from build123d import *

# Parameters (mm, degrees)
BOSS_EXTRUDE1_DEPTH   = 90
BOSS_EXTRUDE1_2_DEPTH = 90
SKETCH3_W             = 2
SKETCH3_H             = 3.026273801
EXTRUDE_THIN1_DEPTH   = 160
SKETCH5_W             = 160
SKETCH5_H             = 110
BOSS_EXTRUDE2_DEPTH   = 5
BOSS_EXTRUDE3_DEPTH   = 5
SKETCH7_W             = 2
SKETCH7_H             = 100
CUT_EXTRUDE1_DEPTH    = 2.5
SKETCH8_W             = 2
SKETCH8_H             = 90
CUT_EXTRUDE2_DEPTH    = 2.5
SKETCH9_W             = 2
SKETCH9_H             = 90
CUT_EXTRUDE3_DEPTH    = 2.5
SKETCH10_W            = 2
SKETCH10_H            = 2.5
CUT_EXTRUDE4_DEPTH    = 2.5
BOSS_EXTRUDE4_DEPTH   = 160
SKETCH12_W            = 100
SKETCH12_H            = 110
BOSS_EXTRUDE5_DEPTH   = 5
FILLET1_R             = 1


with BuildPart() as part:
    # Sketch2 → Boss-Extrude1 (new body)
    with BuildSketch(Plane.XY):
        Polygon((80, 55), (-80, 55), (-80, 50), (-75, 50), (75, 50), (80, 50), align=None)
    extrude(amount=BOSS_EXTRUDE1_DEPTH)



with BuildPart() as body_2:
    # Sketch2 → Boss-Extrude1 2 (new body)
    with BuildSketch(Plane.XY):
        Polygon((-75, -50), (-80, -50), (-80, -55), (80, -55), (80, -50), (75, -50), align=None)
    extrude(amount=BOSS_EXTRUDE1_2_DEPTH)


with BuildPart() as part_1:
    add(part.part)

    add(body_2.part)  # Extrude-Thin1 merges body 2
    # Sketch3 → Extrude-Thin1 (add)
    with BuildSketch(Plane(origin=(80, 0, 0), x_dir=(0, 0, -1), z_dir=(1, 0, 0))):
        with Locations((-36, 48.486863099)):
            Rectangle(SKETCH3_W, SKETCH3_H)
        with Locations((-34, -48.486863099)):
            Rectangle(SKETCH3_W, SKETCH3_H)
        with Locations((-40, 48.486863099)):
            Rectangle(SKETCH3_W, SKETCH3_H)
        with Locations((-38, -48.486863099)):
            Rectangle(SKETCH3_W, SKETCH3_H)
    extrude(amount=-EXTRUDE_THIN1_DEPTH)

    # Sketch5 → Boss-Extrude2 (add)
    with BuildSketch(Plane(origin=(0, 0, 0), x_dir=(-1, 0, 0), z_dir=(0, 0, -1))):
        Rectangle(SKETCH5_W, SKETCH5_H)
    extrude(amount=BOSS_EXTRUDE2_DEPTH)

    # Sketch6 → Boss-Extrude3 (add)
    with BuildSketch(Plane(origin=(80, 0, 0), x_dir=(0, 0, -1), z_dir=(1, 0, 0))):
        Polygon((-90, 55), (-90, 50), (0, 50), (0, -50), (-90, -50), (-90, -55), (5, -55), (5, 55), align=None)
    extrude(amount=BOSS_EXTRUDE3_DEPTH)

    # Sketch7 → Cut-Extrude1 (cut)
    with BuildSketch(Plane.XY):
        with Locations((82.5, 0)):
            Rectangle(SKETCH7_W, SKETCH7_H)
    extrude(amount=-CUT_EXTRUDE1_DEPTH, mode=Mode.SUBTRACT)

    # Sketch8 → Cut-Extrude2 (cut)
    with BuildSketch(Plane.XZ.offset(-50)):
        with Locations((82.5, 45)):
            Rectangle(SKETCH8_W, SKETCH8_H)
    extrude(amount=-CUT_EXTRUDE2_DEPTH, mode=Mode.SUBTRACT)

    # Sketch9 → Cut-Extrude3 (cut)
    with BuildSketch(Plane(origin=(0, -50, 0), x_dir=(1, 0, 0), z_dir=(0, 1, 0))):
        with Locations((82.5, -45)):
            Rectangle(SKETCH9_W, SKETCH9_H)
    extrude(amount=-CUT_EXTRUDE3_DEPTH, mode=Mode.SUBTRACT)

    # Sketch10 → Cut-Extrude4 (cut)
    with BuildSketch(Plane.XY):
        with Locations((82.5, 51.25)):
            Rectangle(SKETCH10_W, SKETCH10_H)
        with Locations((82.5, -51.25)):
            Rectangle(SKETCH10_W, SKETCH10_H)
    extrude(amount=-CUT_EXTRUDE4_DEPTH, mode=Mode.SUBTRACT)

    # Sketch11 → Boss-Extrude4 (add)
    with BuildSketch(Plane.ZY.offset(80)):
        Polygon((90, 50), (90, 55), (95, 55), (95, 50), (93.5, 50), (93.5, 53.5), (91.5, 53.5), (91.5, 50), align=None)
        Polygon((91.5, -53.5), (93.5, -53.5), (93.5, -50), (95, -50), (95, -55), (90, -55), (90, -50), (91.5, -50), align=None)
    extrude(amount=-BOSS_EXTRUDE4_DEPTH)

    # Sketch12 → Boss-Extrude5 (add)
    with BuildSketch(Plane.ZY.offset(80)):
        with Locations((45, 0)):
            Rectangle(SKETCH12_W, SKETCH12_H)
    extrude(amount=BOSS_EXTRUDE5_DEPTH)

    # Fillet1
    fillet1_edges = [part_1.edges().sort_by_distance(p)[0] for p in [
        (80, 52.5, 95),
        (80, -52.5, 95),
        (85, 52.5, 90),
        (85, -52.5, 90),
    ]]
    fillet(fillet1_edges, radius=FILLET1_R)


solid = part_1.part
The model under review builds one solid part; all positions refer to its coordinate system, in mm. A direction names the side the tool comes from. Give positions to 0.01 mm unless a question says otherwise; leave off trailing zeros. Loops run counter-clockwise (first coordinate to the right, second up) from the corner with the lowest first, then second, coordinate; pieces in that order, holes last. Notation, with made-up numbers: (20, 20) -> (59, 20) arc R11 ccw to (59, 27) -> close; hole circle Ø8 at (47.5, 64). An arc over 180 degrees is marked (long way). Put each result on its own line as item: value. Start each with the question number.
1. For faces 1 (the face through (-1, -52, 91.5)), 2 (the face through (80, 53, 91)), 3 (the face through (83.5, 0, -1)), 4 (the face through (1, 55, 44)), list the 3-axis set-ups (+Z, -Z, +X, -X, +Y, -Y) from which the entire face can be reached by the end or side of a thin tool; tool diameter is ignored.
2. Clearance check with flat-ended pins moving along their axes: P1, Ø2, axis at y = 14, z = 39, coming from the +X side; P2, Ø3, axis at y = 52, z = 92, coming from the +X side; P3, Ø1, axis at x = 18, y = 33, coming from the +Z side. State where each tip first meets the part, or that it passes through.
3. Wall thickness on probe 1 along Y at (x, z) = (21.5, 87); probe 2 along X at (y, z) = (-19, 34.5); probe 3 along Z at (x, y) = (-52.5, 6.5): over which ranges is each line inside the solid? List them lowest first.
4. We need section A-A on y = -7.5. State the section outline as (x, z) points, then the cut area to 3 significant figures.
5. We need section B-B on z = 15.5. State the section outline as (x, y) points.
6. Mouldability with a two-part tool opening along Z and no side actions: class faces 5 (the face through (-27, -53, 95)), 6 (the face through (81.5, 0, -1)), 7 (the face through (0, 50, 46)) as released by +Z, released by -Z, zero draft, split by the parting line, or undercut.
Determined:
1. face 1: +X
1. face 2: +Z, +X, +Y, -Y
1. face 3: +Z
1. face 4: +Z, -Z, +X, -X, +Y
2. P1: x = -80
2. P2: x = 80
2. P3: z = 0
3. probe 1: -55 to -50, 50 to 55
3. probe 2: -85 to -80
3. probe 3: -5 to 0
4. outline: (-85, -5) -> (85, -5) -> (85, 0) -> (83.5, 0) -> (83.5, -2.5) -> (81.5, -2.5) -> (81.5, 0) -> (-80, 0) -> (-80, 95) -> (-85, 95) -> close
4. area: 1,320 mm^2
5. outline: (-85, -55) -> (85, -55) -> (85, -50) -> (83.5, -50) -> (83.5, -52.5) -> (81.5, -52.5) -> (81.5, -50) -> (-80, -50) -> (-80, 50) -> (81.5, 50) -> (81.5, 52.5) -> (83.5, 52.5) -> (83.5, 50) -> (85, 50) -> (85, 55) -> (-85, 55) -> close
6. face 5: released by +Z
6. face 6: zero draft
6. face 7: undercut
